The listing builds one solid part. Answer for the finished solid, in the listing's coordinates (mm). Face numbers are marked on the shaded views. Coordinates: 2 decimals unless noted, no trailing zeros. Order: outer loops, then holes, each group sorted by start corner. A loop starts at its lowest first (then second) coordinate and runs counter-clockwise, first axis right, second up. Notation, with made-up numbers: M 67,50.5 L 75,50.5 A22 ccw 75,68.5 Z; hole C 28.5,16.5 d1. An arc over 180 degrees is marked long. One line per item, written item: value. Start each with the question number.
Q1. The part is cut by section B-B on y = -4.5. Give the vertices of the cut face in (x, z).
Q2. The part is cut by section C-C on x = 6. Give the vertices of the cut face in (y, z).
Q3. Straight lines are drawn through the part: line 1 along Y through (x, z) = (-47, 1.45); line 2 along X through (y, z) = (-24.5, 2.55); line 3 along X through (y, z) = (7, 1.6). For each, find the intervals that lie inside material, in ascending order. Write a range as [from, to].
Q4. Each of these flat-tipped pins is pushed along its axis until it touches: pin 1 Ø1.6 at (y, z) = (-4, 3.5) entering from +X; pin 2 Ø2 at (y, z) = (-3.5, 3.5) entering from -X; pin 3 Ø5.5 at (x, y) = (47, 30) entering from -Z; pin 4 Ø2 at (x, y) = (-47.5, -13) entering from +Z. Where does it stop, or does it pass through?
Q5. The part is cut by section A-A on x = 47. Give the vertices of the cut face in (y, z).
Q6. Determine the mould class of the marked faces 1 and 2 for opening direction X: pulls with the +X half, pulls with the -X half, needs draft (parallel to the pull), parting line crosses it, or undercut.
```python
from build123d import *

# Parameters (mm, degrees)
SKETCH_1_W          = 100
SKETCH_1_H          = 72
EXTRUDE_1_DEPTH     = 4
SKETCH_2_W          = 80
SKETCH_2_H          = 65
CUT_EXTRUDE_1_DEPTH = 2
SKETCH_3_R          = 1.65
CUT_EXTRUDE_2_DEPTH = 2
SKETCH_4_R          = 1.65
CUT_EXTRUDE_3_DEPTH = 4
SKETCH_5_W          = 7
SKETCH_5_H          = 72
CUT_EXTRUDE_4_DEPTH = 2
SKETCH_6_W          = 55
SKETCH_6_H          = 50
CUT_EXTRUDE_5_DEPTH = 2


with BuildPart() as part:
    # 草图1 → 凸台-拉伸1 (new body)
    with BuildSketch(Plane.XY):
        Rectangle(SKETCH_1_W, SKETCH_1_H)
    extrude(amount=EXTRUDE_1_DEPTH)

    # 草图2 → 切除-拉伸1 (cut)
    with BuildSketch(Plane.XY.offset(4)):
        Rectangle(SKETCH_2_W, SKETCH_2_H)
    extrude(amount=-CUT_EXTRUDE_1_DEPTH, mode=Mode.SUBTRACT)

    # 草图3 → 切除-拉伸2 (cut)
    with BuildSketch(Plane.XY.offset(2)):
        with Locations((-38.340391641, 30.83641332)):
            Circle(SKETCH_3_R)
        with Locations((38.240608359, 30.83641332)):
            Circle(SKETCH_3_R)
        with Locations((38.240608359, -30.75858668)):
            Circle(SKETCH_3_R)
        with Locations((-38.340391641, -30.75858668)):
            Circle(SKETCH_3_R)
    extrude(amount=-CUT_EXTRUDE_2_DEPTH, mode=Mode.SUBTRACT)

    # 草图4 → 切除-拉伸3 (cut)
    with BuildSketch(Plane.XY.offset(4)):
        with Locations((-47, 30)):
            Circle(SKETCH_4_R)
        with Locations((47, 30)):
            Circle(SKETCH_4_R)
        with Locations((47, -30)):
            Circle(SKETCH_4_R)
        with Locations((-47, -30)):
            Circle(SKETCH_4_R)
    extrude(amount=-CUT_EXTRUDE_3_DEPTH, mode=Mode.SUBTRACT)

    # 草图5 → 切除-拉伸4 (cut)
    with BuildSketch(Plane.XY.offset(4)):
        with Locations((-46.5, 0)):
            Rectangle(SKETCH_5_W, SKETCH_5_H)
        with Locations((46.5, 0)):
            Rectangle(SKETCH_5_W, SKETCH_5_H)
    extrude(amount=-CUT_EXTRUDE_4_DEPTH, mode=Mode.SUBTRACT)

    # 草图6 → 切除-拉伸5 (cut)
    with BuildSketch(Plane.XY.offset(2)):
        Rectangle(SKETCH_6_W, SKETCH_6_H)
    extrude(amount=-CUT_EXTRUDE_5_DEPTH, mode=Mode.SUBTRACT)


solid = part.part
```
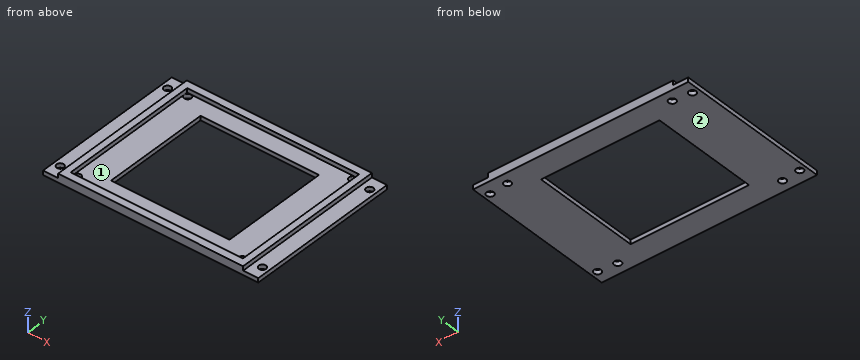
Output:
1. outline: M -50,0 L -27.5,0 L -27.5,2 L -40,2 L -40,4 L -43,4 L -43,2 L -50,2 Z; M 27.5,0 L 50,0 L 50,2 L 43,2 L 43,4 L 40,4 L 40,2 L 27.5,2 Z
2. outline: M -36,0 L -25,0 L -25,2 L -32.5,2 L -32.5,4 L -36,4 Z; M 25,0 L 36,0 L 36,4 L 32.5,4 L 32.5,2 L 25,2 Z
3. line 1: y = [-36, -31.65], [-28.35, 28.35], [31.65, 36]
3. line 2: x = [-43, -40], [40, 43]
3. line 3: x = [-50, -27.5], [27.5, 50]
4. pin 1: stops at x = 43
4. pin 2: stops at x = -43
4. pin 3: stops at z = 0
4. pin 4: stops at z = 2
5. outline: M -36,0 L -31.65,0 L -31.65,2 L -36,2 Z; M -28.35,0 L 28.35,0 L 28.35,2 L -28.35,2 Z; M 31.65,0 L 36,0 L 36,2 L 31.65,2 Z
6. face 1: undercut
6. face 2: needs draft
